Answer from the drawing. Dimensions are ordinates in mm from the lowest x, y and z of the part. A direction names the side the tool comes from. Give positions to 0.01 mm unless a question says otherwise; leave off trailing zeros. Write each loop counter-clockwise with the first axis right and the second up, starting at its lowest first coordinate (ties: lowest second). Pieces come first, ordered by that corner, then holes. Notation, with made-up numbers: (-37, -14) -> (-12, -14) arc R19 cw to (-12, 22) -> close; hole circle Ø6 at (50.25, 14.25). An arc over 180 degrees is marked (long way). Put each result on its own line as item: value. Start each with the question number.
1) Find the intervals of material crossed by line 1 along Z through (x, y) = (18, 7.75); line 2 along Y through (x, z) = (21, 31.5); line 3 along Z through (x, y) = (18, 5.5), in increasing order. Write a range as from..to.
2) A cutting plane is placed at A-A (x = 18). Write down the section's boundary in (y, z), then the cut area to 3 significant figures.
3) A cutting plane is placed at D-D (z = 25). Write down the section's boundary in (x, y), then the cut area to 3 significant figures.
4) A cutting plane is placed at C-C (y = 9.5). Write down the section's boundary in (x, z).
5) For a pull along Z with two mould halves and no side action, classify the marked faces 3, 4 and 5 as released by +Z, released by -Z, zero draft, split by the parting line, or undercut.
6) For the marked faces 1 and 2, determine the directions among +Z, -Z, +X, -X, +Y, -Y from which every point of the face is accessible in a straight line to the end or side of a thin tool.
7) A cutting plane is placed at B-B (z = 18). Write down the section's boundary in (x, y), then the cut area to 3 significant figures.
8) Flat-ended cylindrical pins translate along their axes: pin 1 Ø1.5 at (x, y) = (12, 13) entering from -Z; pin 2 Ø1 at (y, z) = (2.5, 20) entering from +X; pin 3 Ø8 at (x, y) = (19, 9.5) entering from -Z. Find the tip coordinate at first contact, or state that the pin passes through.
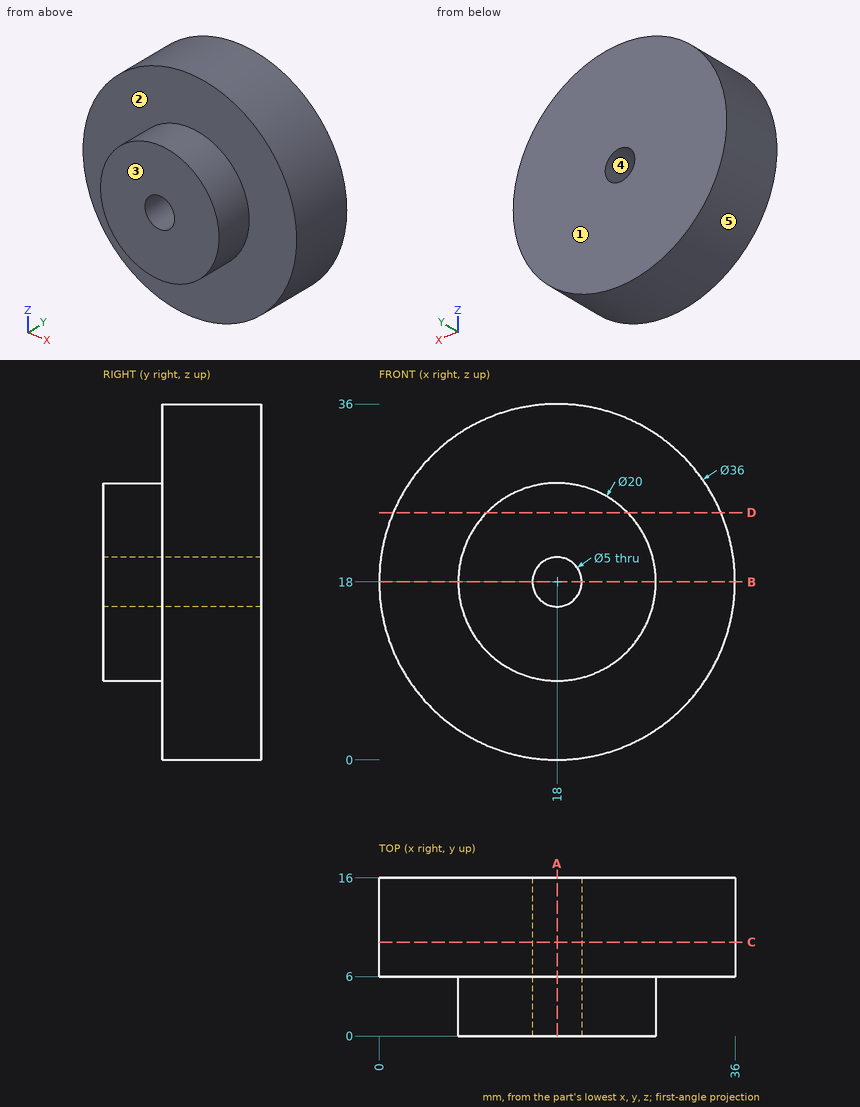
Reply:
1. line 1: z = 0..15.5, 20.5..36
1. line 2: y = 6..16
1. line 3: z = 8..15.5, 20.5..28
2. outline: (0, 8) -> (6, 8) -> (6, 0) -> (16, 0) -> (16, 15.5) -> (0, 15.5) -> close; (0, 20.5) -> (16, 20.5) -> (16, 36) -> (6, 36) -> (6, 28) -> (0, 28) -> close
2. area: 400 mm2
3. outline: (1.42, 6) -> (10.86, 6) -> (10.86, 0) -> (25.14, 0) -> (25.14, 6) -> (34.58, 6) -> (34.58, 16) -> (1.42, 16) -> close
3. area: 417 mm2
4. outline: circle Ø36 at (18, 18); hole circle Ø5 at (18, 18)
5. face 3: zero draft
5. face 4: undercut
5. face 5: split by the parting line
6. face 1: +Z, -Z, +X, -X, +Y
6. face 2: -Y
7. outline: (0, 6) -> (8, 6) -> (8, 0) -> (15.5, 0) -> (15.5, 16) -> (0, 16) -> close; (20.5, 0) -> (28, 0) -> (28, 6) -> (36, 6) -> (36, 16) -> (20.5, 16) -> close
7. area: 400 mm2
8. pin 1: stops at z = 0.78
8. pin 2: stops at x = 27.89
8. pin 3: stops at z = 0
